Could you check a few things on this model? Use its own coordinates, in mm. A direction names the side the tool comes from. Coordinates: 2 decimals unless noted, no trailing zeros. Answer as a JSON object with one key per item and string values. Group by question number.
1) On a 3-axis mill with a long thin cutter (end or side, diameter ignored), from which of +Z, -Z, +X, -X, +Y, -Y can I reach the whole of each face in a straight line? I mean faces 3 (the flat face through (130.708, -13, 44)), 4 (the flat face through (75, -25.4, 64)). Say none if no direction works.
2) If we section it at A-A (y = -13.75): State how many separate pieces and enclosed holes the cut face has, plus the area to 3 significant figures.
3) Please list where these lines run through material, in increasing order: line 1 along Z through (x, y) = (83.5, -23); line 2 along Z through (x, y) = (84.5, -10); line 3 along X through (y, z) = (-6.5, 46).
4) We'd pull the mould along Z, two halves only. Please class faces 1 (the flat face through (74, 0, 64)), 2 (the flat face through (118, -13, 33.261)): released by +Z, released by -Z, zero draft, split by the parting line, or undercut.
5) Will these pins go through, and if not, where does the flat tip stop? pin 1 Ø1.5 at (x, y) = (42.5, -20.5) entering from +Z; pin 2 Ø6 at (x, y) = (63, -8) entering from +Z; pin 3 Ø8 at (x, y) = (19.5, -14.5) entering from +Z.
```python
from build123d import *

# Parameters (mm, degrees)
F0_W     = 152.4
F0_H     = 127.2674917114
F1_DEPTH = 25.4
F1_TAPER = 20
F2_W     = 24.2093652487
F2_H     = 22.6856842637
F3_DEPTH = 25.4
F4_R     = 20.7379881478
F5_DEPTH = 25.4010001


with BuildPart() as f1:
    # F0 (on Front) → F1 (new body)
    with BuildSketch(Plane.XZ):
        with Locations((76.2, 63.6337458557)):
            Rectangle(F0_W, F0_H)
    extrude(amount=F1_DEPTH, taper=F1_TAPER)

    # F2 (on face) → F3 (cut)
    with BuildSketch(Plane.XZ.offset(25.4)):
        with Locations((118.6031028628, 44.6040146053)):
            Rectangle(F2_W, F2_H)
    extrude(amount=-F3_DEPTH, mode=Mode.SUBTRACT)

    # F4 (on face) → F5 (cut, through all)
    with BuildSketch(Plane.XZ.offset(25.4)):
        with Locations((67.5532594323, 97.2846596132)):
            Circle(F4_R)
    extrude(amount=-F5_DEPTH, mode=Mode.SUBTRACT)


solid = f1.part
```
Here are the results:
{
 "1": {"face 3": "+Y, -Y", "face 4": "+Z, -Z, +X, -X, -Y"},
 "2": {"separate pieces": "1", "enclosed holes": "2", "area": "14,800 mm²"},
 "3": {"line 1": "z = 8.37 to 84.03, 110.54 to 118.9", "line 2": "z = 3.64 to 85.33, 109.24 to 123.63", "line 3": "x = 2.37 to 106.5, 130.71 to 150.03"},
 "4": {"face 1": "zero draft", "face 2": "undercut"},
 "5": {"pin 1": "stops at z = 120.08", "pin 2": "stops at z = 125.45", "pin 3": "stops at z = 123.45"}
}
